Could you check a few things on this drawing? It's one solid part, dimensions in mm from its lowest x, y, z. Give positions to 0.01 mm unless a question says otherwise; leave off trailing zeros. Order: outer loops, then holes, each group sorted by start corner. A loop starts at its lowest first (then second) coordinate and runs counter-clockwise, first axis right, second up. Notation, with made-up numbers: (-15, 42) - (2, 42) arc R10 cw to (2, 50) - close; hole circle Ø8 at (29, -21). An arc over 180 degrees is marked (long way). Put each result on its own line as item: value.
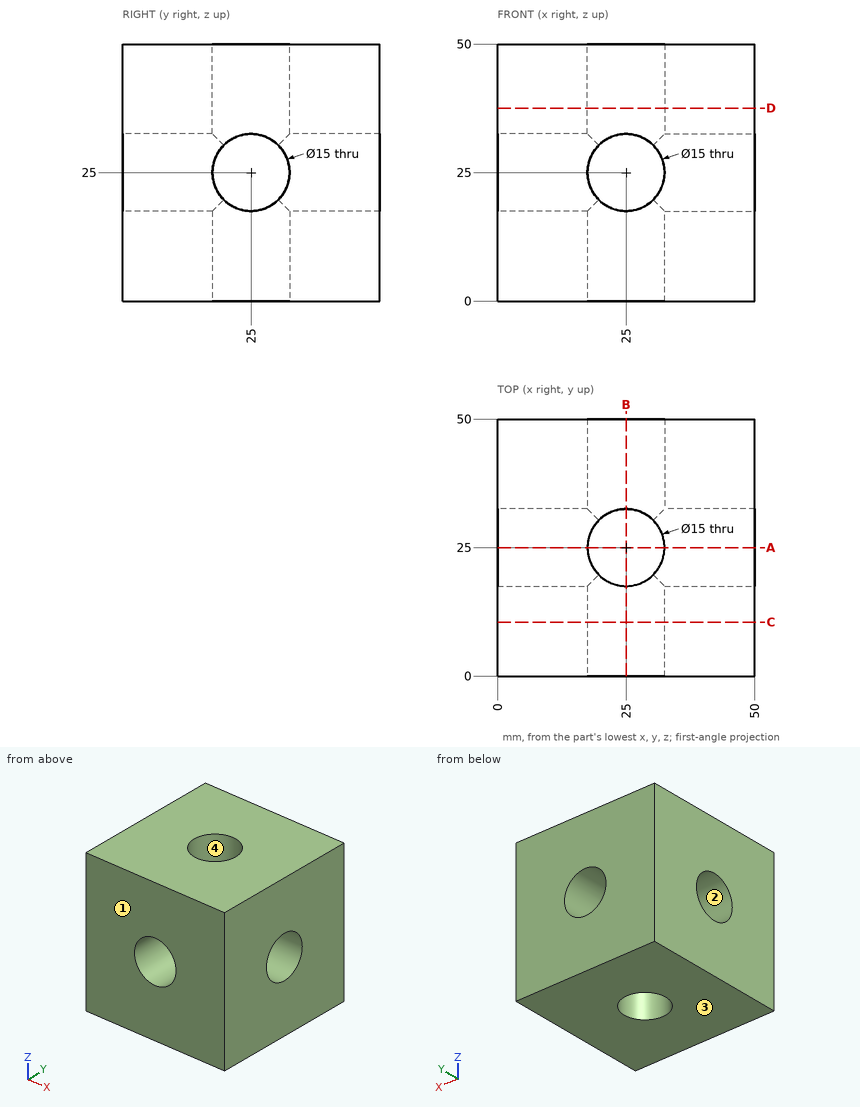
1) If I drill on line 1 (X direction, y = 15.5, z = 25.5); line 2 (Z direction, x = 25, y = 12.25), over which ranges is the centre line in solid material (lowest first)? Write a range as [from, to].
Filled in:
line 1: x = [0, 17.52], [32.48, 50]
line 2: z = [0, 17.5], [32.5, 50]
2) We'd pull the mould along Y, two halves only. Please class the marked faces 1, 2, 3 and 4: pulls with the +Y half, pulls with the -Y half, needs draft (parallel to the pull), parting line crosses it, or undercut.
Filled in:
face 1: pulls with the -Y half
face 2: undercut
face 3: needs draft
face 4: undercut
3) Suppose I cut it at A-A, the plane y = 25. List the corners of the cut face in (x, z) for me.
Filled in:
outline: (0, 0) - (17.5, 0) - (17.5, 17.5) - (0, 17.5) - close; (0, 32.5) - (17.5, 32.5) - (17.5, 50) - (0, 50) - close; (32.5, 0) - (50, 0) - (50, 17.5) - (32.5, 17.5) - close; (32.5, 32.5) - (50, 32.5) - (50, 50) - (32.5, 50) - close
4) I'm going to push a flat-ended pin straight in: pin 1 (12 mm diameter, centred on y = 25, z = 25, fed in from +X). Where does the tip first touch, or does it pass through?
Filled in:
pin 1: passes through
5) Suppose I cut it at C-C, the plane y = 10.5. List the corners of the cut face in (x, z) for me, and give its area (3 significant figures).
Filled in:
outline: (0, 0) - (50, 0) - (50, 50) - (0, 50) - close; hole circle Ø15 at (25, 25)
area: 2,320 mm^2
